Check sheet for the modelled part. Datum: model origin and axes. Units: mm. Round coordinates to 2 decimals unless told otherwise and drop trailing zeros. Loops run counter-clockwise (first coordinate to the right, second up) from the corner with the lowest first, then second, coordinate; pieces in that order, holes last. Notation, with made-up numbers: (86, 42) - (107, 42) arc R25 cw to (107, 76) - close; hole circle Ø2 at (37.5, 71). An arc over 180 degrees is marked (long way). Return JSON: item names as keys, results as strings.
Autodesk Inventor part; units mm, degrees
ref_plane "YZ Plane" through (0, 0, 0) normal (1, 0, 0) x (0, 1, 0)
ref_plane "XZ Plane" through (0, 0, 0) normal (0, 1, 0) x (-1, 0, 0)
ref_plane "XY Plane" through (0, 0, 0) normal (0, 0, 1) x (1, 0, 0)
sketch "Sketch1" plane through (0, 0, 0) normal (0, 0, 1) x (1, 0, 0)
  circle A0 centre (0, 0) radius 3
  circle A1 centre (0, 8) radius 2.25
  circle A2 centre (-8, 0) radius 2.25
  circle A3 centre (0, -8) radius 2.25
  circle A4 centre (8, 0) radius 2.25
  circle A5 centre (0, 0) radius 16
  line L0 (-16, 0) -> (-16, -63.5)
  line L1 (16, 0) -> (16, -63.5)
  line L2 (16, -63.5) -> (-16, -63.5)
  line L3 (0, -63.5) -> (0, 16) construction
  circle A6 centre (-9.65, -57.15) radius 2.25
  circle A7 centre (9.65, -57.15) radius 2.25
  point P0 (-16, -31.75)
  dimension "d0" = 6
  dimension "d1" = 4.5
  dimension "d2" = 8
  dimension "d5" = 360
  dimension "d7" = 32
  dimension "d8" = 63.5
  dimension "d9" = 32
  dimension "d10" = 4.5
  dimension "d11" = 4.5
  dimension "d12" = 6.35
  dimension "d13" = 6.35
  dimension "d14" = 6.35
  dimension "d15" = 6.35
  dimension "d16" = 19.3
extrude "Extrusion1" add sketch "Sketch1" along normal blind 3.175
properties part number "New_Wrist"
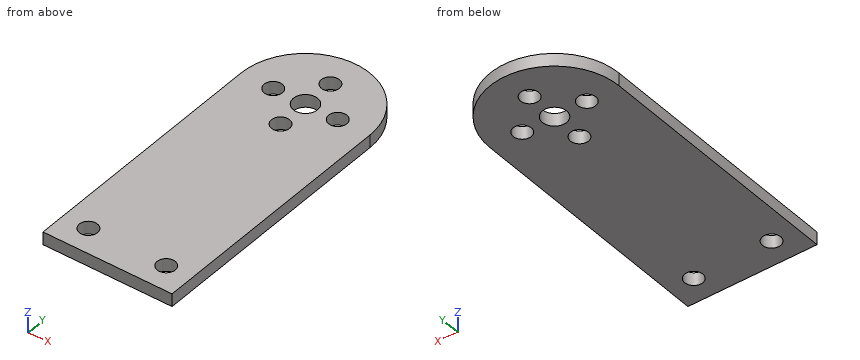
Q1. Sectioned sample at D-D (y = 8). Enter the section's corners in (x, z) (3 decimals), plus the area to 3 significant figures.
Answer key:
{"outline": "(-13.856, 0) - (-2.25, 0) - (-2.25, 3.175) - (-13.856, 3.175) - close; (2.25, 0) - (13.856, 0) - (13.856, 3.175) - (2.25, 3.175) - close", "area": "73.7 mm²"}
Q2. Sectioned sample at A-A (x = 0). Enter the section's corners in (y, z) (3 decimals), plus the area to 3 significant figures.
Answer key:
{"outline": "(-63.5, 0) - (-10.25, 0) - (-10.25, 3.175) - (-63.5, 3.175) - close; (-5.75, 0) - (-3, 0) - (-3, 3.175) - (-5.75, 3.175) - close; (3, 0) - (5.75, 0) - (5.75, 3.175) - (3, 3.175) - close; (10.25, 0) - (16, 0) - (16, 3.175) - (10.25, 3.175) - close", "area": "205 mm²"}
Q3. Scan lines: probe 1 along Y at (x, z) = (0, 1.2); probe 2 along Y at (x, z) = (-10, 1.9); probe 3 along Y at (x, z) = (-11, 0.35). Record each from-to range of solid material in increasing order. Write a range as [from, to].
Answer key:
{"probe 1": "y = [-63.5, -10.25], [-5.75, -3], [3, 5.75], [10.25, 16]", "probe 2": "y = [-63.5, -59.37], [-54.93, -1.03], [1.03, 12.49]", "probe 3": "y = [-63.5, -58.95], [-55.35, 11.62]"}
Q4. Sectioned sample at C-C (x = 11). Enter the section's corners in (y, z) (3 decimals).
Answer key:
{"outline": "(-63.5, 0) - (-58.95, 0) - (-58.95, 3.175) - (-63.5, 3.175) - close; (-55.35, 0) - (11.619, 0) - (11.619, 3.175) - (-55.35, 3.175) - close"}
Q5. Depth check by flat-ended pin: P1, Ø4, axis at x = 8, y = 0, coming from the +Z side. Enter the tip coordinate at first touch or a pass-through.
Answer key:
{"P1": "passes through"}
Q6. Sectioned sample at B-B (z = 0.8). Enter the section's corners in (x, y).
Answer key:
{"outline": "(-16, -63.5) - (16, -63.5) - (16, 0) arc R16 ccw to (-16, 0) - close; hole circle Ø4.5 at (-9.65, -57.15); hole circle Ø4.5 at (-8, 0); hole circle Ø6 at (0, 0); hole circle Ø4.5 at (0, -8); hole circle Ø4.5 at (0, 8); hole circle Ø4.5 at (8, 0); hole circle Ø4.5 at (9.65, -57.15)"}
